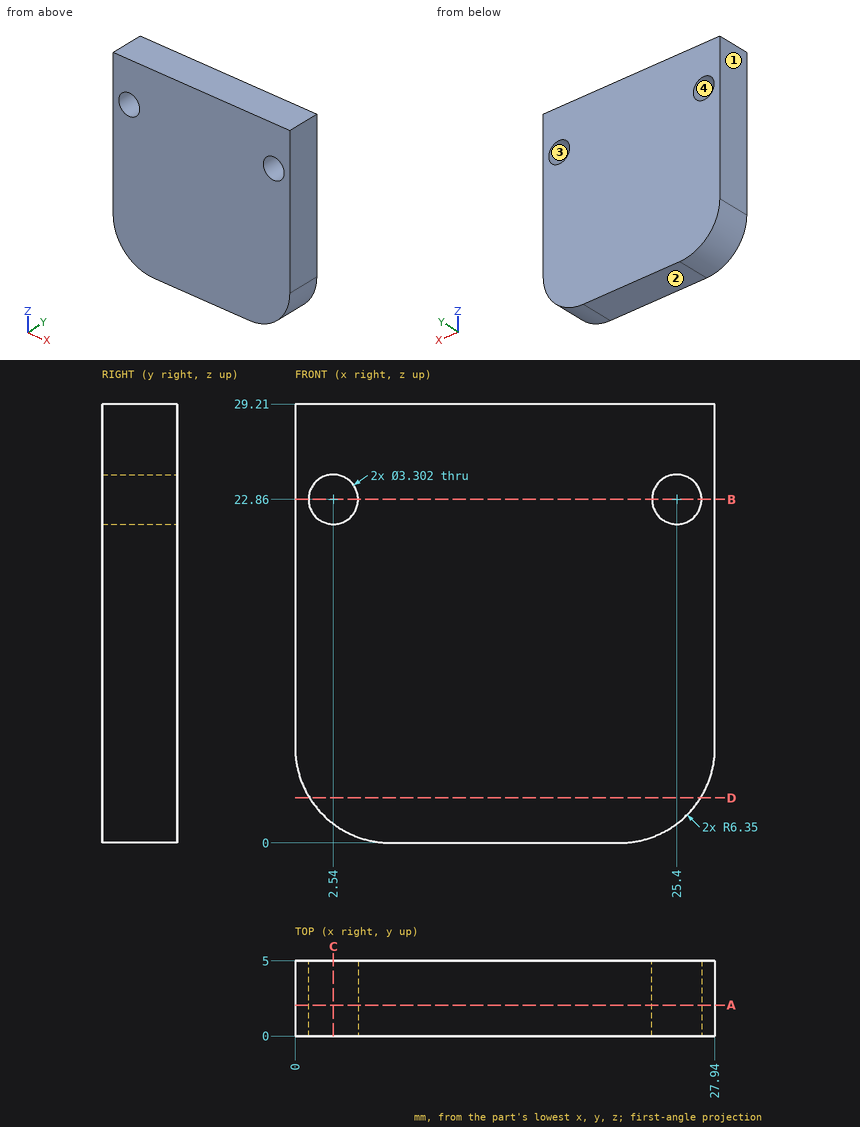
Input: dimensioned drawing with shaded views. Units: mm. Origin: part minimum x, y, z. Give positions to 0.01 mm unless a question says otherwise; leave off trailing zeros. Write each loop counter-clockwise with the first axis right and the second up, starting at its lowest first coordinate (ties: lowest second). Pieces come first, ordered by that corner, then holes. Notation, with made-up numbers: M 32,-24.5 L 89,-24.5 A21 ccw 89,-1.5 Z; hole C 63.5,-29.5 d1. An arc over 180 degrees is marked long. Return JSON: item names as keys, results as strings. Group by question number.
1) Cut plane D-D, the plane z = 3. Output: boundary loops of the cut face in (x, y), plus the area to 3 significant figures.
2) Cut plane B-B, the plane z = 22.86. Output: boundary loops of the cut face in (x, y), plus the area to 3 significant figures.
3) Cut plane C-C, the plane x = 2.54. Output: boundary loops of the cut face in (y, z).
4) Pull-direction query (X, two-part tool) for the marked faces 1, 2, 3 and 4; classes: pulls with the +X half, pulls with the -X half, needs draft (parallel to the pull), parting line crosses it, or undercut.
5) Cut plane A-A, the plane y = 2.05. Output: boundary loops of the cut face in (x, z).
6) Material intervals for line 1 along Z through (x, y) = (25.4, 2.6); line 2 along Z through (x, y) = (6.25, 1.4); line 3 along Z through (x, y) = (5.5, 3.35), sorted ascending. Write a range as [from, to].
Recorded:
{
 "1": {"outline": "M 0.96,0 L 26.98,0 L 26.98,5 L 0.96,5 Z", "area": "130 mm²"},
 "2": {"outline": "M 0,0 L 0.89,0 L 0.89,5 L 0,5 Z; M 4.19,0 L 23.75,0 L 23.75,5 L 4.19,5 Z; M 27.05,0 L 27.94,0 L 27.94,5 L 27.05,5 Z", "area": "107 mm²"},
 "3": {"outline": "M 0,1.27 L 5,1.27 L 5,21.21 L 0,21.21 Z; M 0,24.51 L 5,24.51 L 5,29.21 L 0,29.21 Z"},
 "4": {"face 1": "pulls with the -X half", "face 2": "needs draft", "face 3": "undercut", "face 4": "undercut"},
 "5": {"outline": "M 0,6.35 A6.35 ccw 6.35,0 L 21.59,0 A6.35 ccw 27.94,6.35 L 27.94,29.21 L 0,29.21 Z; hole C 2.54,22.86 d3.3; hole C 25.4,22.86 d3.3"},
 "6": {"line 1": "z = [1.27, 21.21], [24.51, 29.21]", "line 2": "z = [0, 29.21]", "line 3": "z = [0.06, 29.21]"}
}
